Could you check a few things on this model? Use its own coordinates, in mm. Face numbers are marked on the shaded views. Coordinates: 2 decimals unless noted, no trailing zeros. Write each loop counter-clockwise with the first axis right and the second up, starting at its lowest first coordinate (ties: lowest second). Pieces come first, ordered by that corner, then holes.
Item 1: I want a section at C-C on x = 5. Please give me the cut outline in (y, z) (3 decimals), then the cut area to 3 significant figures.
Item 2: I want a section at A-A on y = 0. State how many separate pieces and enclosed holes the cut face has, then the cut area to 3 significant figures.
Item 3: If I drill on probe 1 along Z at (x, y) = (0, -10.2); probe 2 along Y at (x, z) = (-0.5, 20); probe 3 along Z at (x, y) = (7, -5.25), over which ranges is the centre line in solid material (lowest first)?
Item 4: Thinking about a two-plate mould opening in Y: for the marked faces 1, 2 and 3, which applies, +Y half, -Y half, draft (parallel to the pull), parting line (faces both ways), or undercut?
Item 5: For P1, Ø3.5, axis at y = 0, z = 15, coming from the -X side; P2, Ø6, axis at x = -2, y = -5.5, coming from the -Z side; P3, Ø2, axis at y = 8.5, z = 32, coming from the +X side; P4, Ø1.8, axis at x = 0, z = 15, coming from the -Y side, each with a flat end and sliding along its axis, tell me the tip position at first contact or that it passes through.
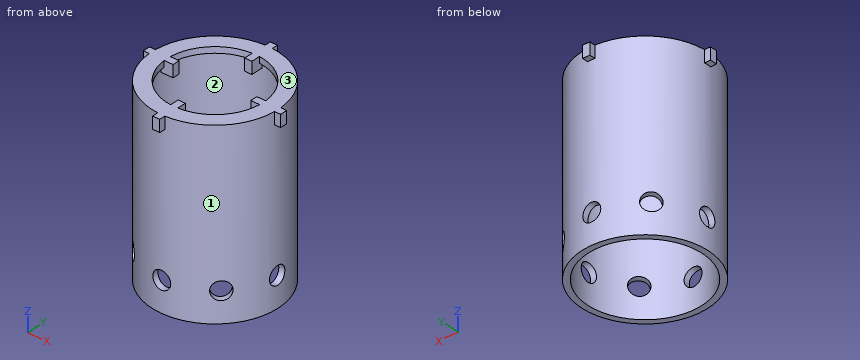
from build123d import *

# Parameters (mm, degrees)
EXTRUDE_START            = 10
SKETCH_1_R               = 10.5
SKETCH_1_R_2             = 9.5
EXTRUDE_1_DEPTH          = 30
EXTRUDE_START_2          = 40
SKETCH_6_R               = 10
SKETCH_6_R_2             = 8
EXTRUDE_3_DEPTH          = 1
SKETCH_5_W               = 2
SKETCH_5_H               = 1.2
EXTRUDE_4_DEPTH          = 2
PATTERN_CIRCULAR_1_COUNT = 4
SKETCH_7_R               = 1.5
CUT_EXTRUDE_2_DEPTH      = 20
PATTERN_CIRCULAR_2_COUNT = 8


with BuildPart() as part:
    # ｽｹｯﾁ1 → ﾎﾞｽ - 押し出し1 (new body)
    with BuildSketch(Plane.XY.offset(EXTRUDE_START)):
        Circle(SKETCH_1_R)
        Circle(SKETCH_1_R_2, mode=Mode.SUBTRACT)
    extrude(amount=EXTRUDE_1_DEPTH)

    # ｽｹｯﾁ6 → ﾎﾞｽ - 押し出し3 (add)
    with BuildSketch(Plane.XY.offset(EXTRUDE_START_2)):
        Circle(SKETCH_6_R)
        Circle(SKETCH_6_R_2, mode=Mode.SUBTRACT)
    extrude(amount=-EXTRUDE_3_DEPTH)

    # ｽｹｯﾁ5 → ﾎﾞｽ - 押し出し4 (add)
    with BuildSketch(Plane.XY.offset(40)):
        with Locations((7.5, 0)):
            Rectangle(SKETCH_5_W, SKETCH_5_H)
        with Locations((10.48172138, -0.010967172)):
            Rectangle(SKETCH_5_W, SKETCH_5_H)
    extrude_4 = extrude(amount=-EXTRUDE_4_DEPTH)

    # 円形ﾊﾟﾀｰﾝ1: ﾎﾞｽ - 押し出し4 ×4 about axis
    pattern_circular_1_axis = Axis((0, 0, 0), (0, 0, 1))
    for i in range(1, PATTERN_CIRCULAR_1_COUNT):
        add(extrude_4.rotate(pattern_circular_1_axis, i * 360 / PATTERN_CIRCULAR_1_COUNT))

    # ｽｹｯﾁ7 → ｶｯﾄ - 押し出し2 (cut, symmetric)
    with BuildSketch(Plane(origin=(0, 0, 0), x_dir=(0, 0, -1), z_dir=(1, 0, 0))):
        with Locations((-15, 0)):
            Circle(SKETCH_7_R)
    cut_extrude_2 = extrude(amount=CUT_EXTRUDE_2_DEPTH, both=True, mode=Mode.SUBTRACT)

    # 円形ﾊﾟﾀｰﾝ2: ｶｯﾄ - 押し出し2 ×8 about axis
    pattern_circular_2_axis = Axis((0, 0, 39), (0, 0, 1))
    for i in range(1, PATTERN_CIRCULAR_2_COUNT):
        add(cut_extrude_2.rotate(pattern_circular_2_axis, i * 360 / PATTERN_CIRCULAR_2_COUNT), mode=Mode.SUBTRACT)


solid = part.part
Response values:
1. outline: (-9.233, 10) - (-8.078, 10) - (-8.078, 39) - (-6.245, 39) - (-6.245, 40) - (-9.233, 40) - close; (6.245, 39) - (8.078, 39) - (8.078, 10) - (9.233, 10) - (9.233, 40) - (6.245, 40) - close
1. area: 73.0 mm2
2. separate pieces: 4
2. enclosed holes: 0
2. area: 68.0 mm2
3. probe 1: z = 10 to 13.5, 16.5 to 40
3. probe 2: y = -10.49 to -9.49, 9.49 to 10.49
3. probe 3: z = 39 to 40
4. face 1: parting line
4. face 2: undercut
4. face 3: draft
5. P1: stops at x = -10.5
5. P2: stops at z = 38
5. P3: stops at x = 7.35
5. P4: passes through
